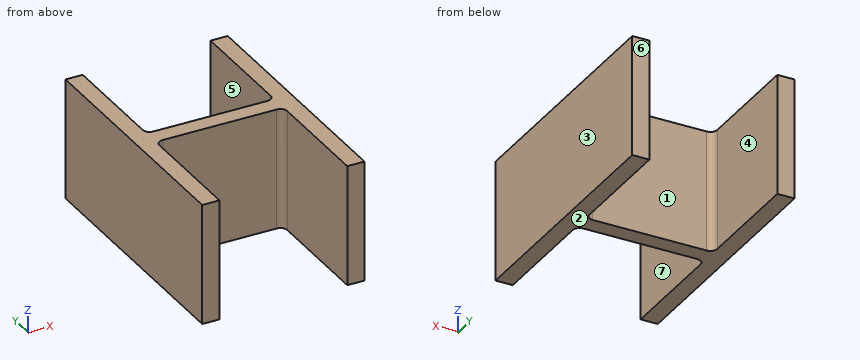
Autodesk Inventor part; units mm, degrees
ref_plane "YZ Plane" through (0, 0, 0) normal (1, 0, 0) x (0, 1, 0)
ref_plane "XZ Plane" through (0, 0, 0) normal (0, 1, 0) x (-1, 0, 0)
ref_plane "XY Plane" through (0, 0, 0) normal (0, 0, 1) x (1, 0, 0)
sketch "Sketch1" plane through (0, 0, 0) normal (0, 1, 0) x (-1, 0, 0)
  line L0 (0, 0) -> (47.1, 0)
  line L1 (47.1, 0) -> (47.1, -35)
  line L2 (47.1, -35) -> (0, -35)
  line L3 (0, -35) -> (0, 0)
  line L4 (47.1, 0) -> (42.1, 0)
  line L5 (42.1, 0) -> (42.1, -35)
  line L6 (42.1, -35) -> (47.1, -35)
  line L7 (47.1, -35) -> (47.1, 0)
  line L8 (42.1, -15) -> (5, -15)
  line L9 (0, -11) -> (0, -16)
  line L10 (5, -20) -> (42.1, -20)
  line L11 (42.1, -20) -> (42.1, -15)
  line L12 (0, 0) -> (5, 0)
  line L13 (5, 0) -> (5, -35)
  line L14 (5, -35) -> (0, -35)
  line L15 (0, -35) -> (0, 0)
  dimension "d0" = 47.1
  dimension "d1" = 35
  dimension "d2" = 5
  dimension "d3" = 5
  dimension "d4" = 15
  dimension "d6" = 5
  dimension "d7" = 35
  dimension "d15" = 15
extrude "Extrusion1" add sketch "Sketch1" along normal blind 73.5 contours L0 L13 L2 L3 | L0 L1 L2 L5
sketch "Sketch2" plane through (-47.1, 0, 0) normal (0, 0, 1) x (1, 0, 0)
  line L0 (0, 0) -> (5, 0)
  line L1 (5, 0) -> (5, 73.5)
  line L2 (0, 73.5) -> (5, 73.5)
  line L3 (0, 0) -> (0, 73.5)
  line L4 (42.1, 0) -> (47.1, 0)
  line L5 (47.1, 0) -> (47.1, 73.5)
  line L6 (42.1, 73.5) -> (47.1, 73.5)
  line L7 (42.1, 0) -> (42.1, 73.5)
  line L8 (5, 0) -> (5, 73.5)
  line L9 (42.1, 0) -> (42.1, 73.5)
  line L10 (42.1, 15.5) -> (42.1, 10.5)
  line L11 (5, 10.5) -> (5, 15.5)
  line L12 (47.1, 0) -> (47.1, 73.5)
  line L13 (0, 0) -> (0, 73.5)
  line L14 (47.1, 39.25) -> (0, 39.25)
  line L15 (0, 39.25) -> (0, 34.25)
  line L16 (0, 34.25) -> (47.1, 34.25)
  line L17 (47.1, 34.25) -> (47.1, 39.25)
  dimension "d10" = 5
  dimension "d16" = 5
  dimension "d17" = 34.25
sketch "Sketch3" plane through (0, 0, 0) normal (0, -1, 0) x (1, 0, 0)
  line L0 (-43.6752, -16.6981) -> (-43.6752, -10.5412) construction
  line L1 (-43.6752, -10.5412) -> (-38.9883, -10.5412) construction
  line L2 (-38.9883, -10.5412) -> (-38.9883, -16.6981) construction
  line L3 (-38.9883, -16.6981) -> (-43.6752, -16.6981) construction
  point P0 (0, 0)
extrude "Extrusion3" add sketch "Sketch2" against normal blind 35 contours L3 L14 L1 L16 | L1 L14 L7 L16 | L7 L14 L5 L16
fillet "Fillet2" radius 2 4 edges at (-5, 34.25, -17.5) (-42.1, 34.25, -17.5) (-5, 39.25, -17.5) (-42.1, 39.25, -17.5)
properties part number "150x0y0z_0x0y0z"
The listing builds one solid part. Answer for the finished solid, in the listing's coordinates (mm). Face numbers are marked on the shaded views. A direction names the side the tool comes from. Give positions to 0.01 mm unless a question says otherwise; leave off trailing zeros. Write each loop counter-clockwise with the first axis right and the second up, starting at its lowest first coordinate (ties: lowest second). Pieces come first, ordered by that corner, then holes. Notation, with made-up numbers: (52, 8.25) -> (70, 8.25) arc R19 ccw to (70, 40.25) -> close; hole circle Ø5 at (52, 32). An arc over 180 degrees is marked (long way). Use a Markdown table: item, result.
(1) Flat-ended cylindrical pins translate along their axes: P1, Ø8, axis at x = -18, z = -6.5, coming from the -Y side; P2, Ø1, axis at x = -26, z = -21, coming from the +Y side; P3, Ø1.5, axis at x = -6.5, z = -8.5, coming from the +Y side. Find the tip coordinate at first contact, or state that the pin passes through.
Return value:
| item | result |
|---|---|
| P1 | y = 34.25 |
| P2 | y = 39.25 |
| P3 | y = 39.69 |
(2) Determine the mould class of the marked faces 1, 2, 3 and 4 for opening direction X: released by +X, released by -X, zero draft, split by the parting line, or undercut.
Return value:
| item | result |
|---|---|
| face 1 | undercut |
| face 2 | zero draft |
| face 3 | released by +X |
| face 4 | undercut |
(3) Section A-A, the plane y = 21 is taken. Determine the outline of the cut face in (x, z), then the cut area to 3 significant figures.
Return value:
| item | result |
|---|---|
| outline | (-47.1, -35) -> (-42.1, -35) -> (-42.1, 0) -> (-47.1, 0) -> close; (-5, -35) -> (0, -35) -> (0, 0) -> (-5, 0) -> close |
| area | 350 mm2 |
(4) Section C-C, the plane x = -33.5 is taken. Determine the outline of the cut face in (y, z), then the cut area to 3 significant figures.
Return value:
| item | result |
|---|---|
| outline | (34.25, -35) -> (39.25, -35) -> (39.25, 0) -> (34.25, 0) -> close |
| area | 175 mm2 |
(5) Section B-B, the plane z = -30.5 is taken. Determine the outline of the cut face in (x, y), then the cut area to 3 significant figures.
Return value:
| item | result |
|---|---|
| outline | (-47.1, 0) -> (-42.1, 0) -> (-42.1, 32.25) arc R2 cw to (-40.1, 34.25) -> (-7, 34.25) arc R2 cw to (-5, 32.25) -> (-5, 0) -> (0, 0) -> (0, 73.5) -> (-5, 73.5) -> (-5, 41.25) arc R2 cw to (-7, 39.25) -> (-40.1, 39.25) arc R2 cw to (-42.1, 41.25) -> (-42.1, 73.5) -> (-47.1, 73.5) -> close |
| area | 924 mm2 |
(6) Find the intervals of material crossed by probe 1 along X at (y, z) = (44, -18); probe 2 along Y at (x, z) = (-27, -16), in increasing order. Write a range as from..to.
Return value:
| item | result |
|---|---|
| probe 1 | -47.1..-42.1, -5..0 |
| probe 2 | 34.25..39.25 |
(7) For the marked faces 5, 6 and 7, determine the directions among +Z, -Z, +X, -X, +Y, -Y from which every point of the face is accessible in a straight line to the end or side of a thin tool.
Return value:
| item | result |
|---|---|
| face 5 | +Z, -Z, +Y |
| face 6 | +Z, -Z, +X, -X, +Y |
| face 7 | +Z, -Z, -Y |
